The model under review builds one solid part; all positions refer to its coordinate system, in mm. A direction names the side the tool comes from. Coordinates: 2 decimals unless noted, no trailing zeros. Write each loop counter-clockwise with the first axis right and the second up, starting at its lowest first coordinate (ties: lowest second). Pieces come first, ordered by that corner, then holes. Notation, with made-up numbers: (-1.5, -25) - (13.5, -25) arc R22 ccw to (13.5, -8) - close; hole circle Ø2 at (-31, 4). An arc over 180 degrees is marked (long way). Use one line per item in the form item = value. Start each with the question number.
```python
from build123d import *

# Parameters (mm, degrees)
BOSS_EXTRUDE1_DEPTH      = 2
BOSS_EXTRUDE2_DEPTH      = 2
BOSS_EXTRUDE2_DEPTH_BACK = 2
SKETCH2_W                = 2
SKETCH2_H                = 15
SKETCH3_R                = 1
CUT_EXTRUDE1_DEPTH       = 25.320588628


with BuildPart() as part:
    # Sketch1 → Boss-Extrude1 (new body)
    with BuildSketch(Plane(origin=(0, 0, 0), x_dir=(1, 0, 0), z_dir=(0, 1, 0))):
        with BuildLine():
            Line((3.889087297, -3.889087297), (5.303300859, -5.303300859))
            ThreePointArc((5.303300859, -5.303300859), (0, 7.5), (-5.303300859, -5.303300859))
            Line((-5.303300859, -5.303300859), (-3.889087297, -3.889087297))
            ThreePointArc((-3.889087297, -3.889087297), (0, 5.5), (3.889087297, -3.889087297))
        make_face()
    extrude(amount=BOSS_EXTRUDE1_DEPTH)

    # Sketch2 → Boss-Extrude2 (add, two sides: drawn at the far end of the back side and taken through both)
    with BuildSketch(Plane(origin=(0, 2, 0), x_dir=(1, 0, 0), z_dir=(0, 1, 0)).offset(-BOSS_EXTRUDE2_DEPTH_BACK)):
        with Locations((0, 14.933034374)):
            Rectangle(SKETCH2_W, SKETCH2_H)
    extrude(amount=BOSS_EXTRUDE2_DEPTH + BOSS_EXTRUDE2_DEPTH_BACK)

    # Sketch3 → Cut-Extrude1 (cut, through all)
    with BuildSketch(Plane(origin=(1, 0, 0), x_dir=(0, 0, -1), z_dir=(1, 0, 0))):
        with Locations((16.183034374, 2.5)):
            Circle(SKETCH3_R)
    extrude(amount=-CUT_EXTRUDE1_DEPTH, mode=Mode.SUBTRACT)


solid = part.part
```
1. For P1, Ø2, axis at y = 1.5, z = -12.5, coming from the +X side; P2, Ø2, axis at y = 1, z = -16, coming from the -X side; P3, Ø1, axis at x = -2, y = 1, coming from the +Z side, all flat-tipped, find the tip position at first contact; note any pin that passes through.
2. For L1, parallel to X at y = 0.7, z = 0; L2, parallel to X at y = 1.75, z = -7.5; L3, parallel to Z at x = 4, y = 0.4, list the stretches that pass through material, from the lowest coordinate up.
3. Take a section at B-B (y = 2.5). State the section outline as (x, z) points.
4. The part is to be moulded in two halves that separate along Y. For faces 1 (the flat face through (0, 0, -6)), 2 (the flat face through (0, 2, -22.433)), 3 (the flat face through (1, 2, -6)), 4 (the cylindrical face through (0.014, 2.544, -15.184)), say which applies: released by +Y, released by -Y, zero draft, split by the parting line, or undercut.
5. For faces 5 (the flat face through (1, 2, -15)), 6 (the flat face through (0, 3, -7.433)), 7 (the flat face through (-5, 1, 5)), 8 (the flat face through (-1, 2, -15)), list the 3-axis set-ups (+Z, -Z, +X, -X, +Y, -Y) from which the entire face can be reached by the end or side of a thin tool; tool diameter is ignored.
6. Take a section at D-D (z = -20.5). State the section outline as (x, y) points, plus the area to 3 significant figures.
7. Take a section at C-C (x = 0). State the section outline as (y, z) points, plus the area to 3 significant figures.
8. Take a section at A-A (z = 0). State the section outline as (x, y) points.
Returned:
q1.P1 = 1
q1.P2 = -1
q1.P3 = -4.9
q2.L1 = -7.5 to -5.5, 5.5 to 7.5
q2.L2 = -1 to 1
q2.L3 = -6.34 to -3.77, 3.77 to 4
q3.outline = (-1, -22.43) - (1, -22.43) - (1, -17.18) - (-1, -17.18) - close; (-1, -15.18) - (1, -15.18) - (1, -7.43) - (-1, -7.43) - close
q4.face_1 = released by -Y
q4.face_2 = zero draft
q4.face_3 = released by +Y
q4.face_4 = undercut
q5.face_5 = -Z, +X, +Y, -Y
q5.face_6 = +Z, +X, -X, +Y
q5.face_7 = +Z, +Y, -Y
q5.face_8 = -Z, -X, +Y, -Y
q6.outline = (-1, 0) - (1, 0) - (1, 4) - (-1, 4) - close
q6.area = 8.00 mm²
q7.outline = (0, -22.43) - (4, -22.43) - (4, -7.43) - (2, -7.43) - (2, -5.5) - (0, -5.5) - close; hole circle Ø2 at (2.5, -16.18)
q7.area = 60.7 mm²
q8.outline = (-7.5, 0) - (-5.5, 0) - (-5.5, 2) - (-7.5, 2) - close; (5.5, 0) - (7.5, 0) - (7.5, 2) - (5.5, 2) - close
